from build123d import *

# Parameters (mm, degrees)
CROQUIS1_W              = 96
CROQUIS1_H              = 67
SALIENTE_EXTRUIR1_DEPTH = 3
CROQUIS2_R              = 2.5
CROQUIS2_R_2            = 4.5
CROQUIS2_R_3            = 1.625
CROQUIS2_W              = 12
CROQUIS2_H              = 12
CROQUIS2_W_2            = 3
CROQUIS2_H_2            = 3
CORTAR_EXTRUIR1_DEPTH   = 59.611005792


with BuildPart() as part:
    # Croquis1 → Saliente-Extruir1 (new body)
    with BuildSketch(Plane.XY):
        Rectangle(CROQUIS1_W, CROQUIS1_H)
    extrude(amount=SALIENTE_EXTRUIR1_DEPTH)

    # Croquis2 → Cortar-Extruir1 (cut, through all)
    with BuildSketch(Plane.XY):
        with Locations((-37.5, 19)):
            Circle(CROQUIS2_R)
        with Locations((-2.5, -8)):
            Circle(CROQUIS2_R_2)
        with Locations((0, 30.5)):
            Circle(CROQUIS2_R_3)
        with Locations((0, -27.5)):
            Circle(CROQUIS2_R_3)
        with Locations((31.5, -8)):
            Rectangle(CROQUIS2_W, CROQUIS2_H)
        with Locations((21, -8)):
            Rectangle(CROQUIS2_W_2, CROQUIS2_H_2)
        with Locations((42, -8)):
            Rectangle(CROQUIS2_W_2, CROQUIS2_H_2)
    extrude(amount=CORTAR_EXTRUIR1_DEPTH, mode=Mode.SUBTRACT)


solid = part.part
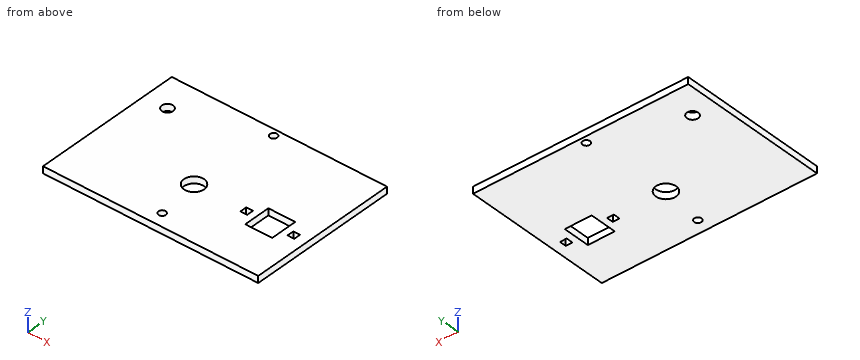
Input: part model. Units: mm. Frame: model coordinates. Coordinates: 2 decimals unless noted, no trailing zeros. Loops run counter-clockwise (first coordinate to the right, second up) from the corner with the lowest first, then second, coordinate; pieces in that order, holes last. Notation, with made-up numbers: (56, -33.75) - (62, -33.75) arc R26 cw to (62, -1.75) - close; hole circle Ø11 at (44.5, 18). An arc over 180 degrees is marked (long way). Answer in a Markdown table with one row per item. Add a question column.
Item 1: Line query: line 1 along X through (y, z) = (-8, 1.5); line 2 along X through (y, z) = (30.5, 1.6) (3 decimals); line 3 along Y through (x, z) = (-2.5, 1.25). Output: solid intervals per line, ascending. Write a range as [from, to].
Item 2: Section query A-A on y = -8. Return the cut outline in (x, z).
Item 3: Section query C-C on z = 2.5. Return the cut outline in (x, y) (3 decimals), then the cut area to 3 significant figures.
Item 4: Contact query for a flat-ended pin moving along its axis: P1, Ø4, axis at x = 0, y = -27.5, coming from the +Z side. Output: stop coordinate, or through.
Item 5: Section query B-B on x = 27. Return the cut outline in (y, z).
Item 6: Section query D-D on y = 30.5. Return the cut outline in (x, z) (3 decimals), then the cut area to 3 significant figures.
Recorded:
| question | item | result |
|---|---|---|
| 1 | line 1 | [-48, -7], [2, 19.5], [22.5, 25.5], [37.5, 40.5], [43.5, 48] |
| 1 | line 2 | [-48, -1.625], [1.625, 48] |
| 1 | line 3 | [-33.5, -12.5], [-3.5, 33.5] |
| 2 | outline | (-48, 0) - (-7, 0) - (-7, 3) - (-48, 3) - close; (2, 0) - (19.5, 0) - (19.5, 3) - (2, 3) - close; (22.5, 0) - (25.5, 0) - (25.5, 3) - (22.5, 3) - close; (37.5, 0) - (40.5, 0) - (40.5, 3) - (37.5, 3) - close; (43.5, 0) - (48, 0) - (48, 3) - (43.5, 3) - close |
| 3 | outline | (-48, -33.5) - (48, -33.5) - (48, 33.5) - (-48, 33.5) - close; hole circle Ø5 at (-37.5, 19); hole circle Ø9 at (-2.5, -8); hole circle Ø3.25 at (0, -27.5); hole circle Ø3.25 at (0, 30.5); hole (19.5, -9.5) - (22.5, -9.5) - (22.5, -6.5) - (19.5, -6.5) - close; hole (25.5, -14) - (37.5, -14) - (37.5, -2) - (25.5, -2) - close; hole (40.5, -9.5) - (43.5, -9.5) - (43.5, -6.5) - (40.5, -6.5) - close |
| 3 | area | 6,170 mm^2 |
| 4 | P1 | z = 3 |
| 5 | outline | (-33.5, 0) - (-14, 0) - (-14, 3) - (-33.5, 3) - close; (-2, 0) - (33.5, 0) - (33.5, 3) - (-2, 3) - close |
| 6 | outline | (-48, 0) - (-1.625, 0) - (-1.625, 3) - (-48, 3) - close; (1.625, 0) - (48, 0) - (48, 3) - (1.625, 3) - close |
| 6 | area | 278 mm^2 |
